Work out the finished part from the listing and answer in its coordinate system (mm). A direction names the side the tool comes from. Coordinates: 2 decimals unless noted, no trailing zeros. Order: outer loops, then holes, each group sorted by start corner. A loop starts at its lowest first (then second) coordinate and runs counter-clockwise, first axis right, second up.
1. Flat-ended cylindrical pins translate along their axes: pin 1 Ø4 at (x, y) = (41.5, -9.5) entering from -Z; pin 2 Ø6 at (y, z) = (-5.5, -31) entering from +X; pin 3 Ø3 at (y, z) = (-10.5, -51.5) entering from -X. Find the tip coordinate at first contact, or state that the pin passes through.
2. Find the intervals of material crossed by probe 1 along X at (y, z) = (2.8, -8); probe 2 along X at (y, z) = (1.4, -62); probe 3 along Z at (x, y) = (7, 2.5), in increasing order.
3. The part is cut by section A-A, the plane z = -62. Give the vertices of the cut face in (x, y).
4. The part is cut by section B-B, the plane z = -41. Give the vertices of the cut face in (x, y).
5. Determine the mould class of faces 4 (the cylindrical face through (25, 2, -37.6)), 5 (the flat face through (35, 4, -32)), 6 (the flat face through (66.05, -6, -11)) for opening direction X: +X half, -X half, draft (parallel to the pull), parting line (faces both ways), or undercut.
6. The part is cut by section C-C, the plane x = 3. Give the vertices of the cut face in (y, z), then the cut area to 3 significant figures.
7. The part is cut by section D-D, the plane y = 2.5. Count the separate pieces of the cut face and the enclosed holes in it, then the cut area to 3 significant figures.
8. A tool of negligible diameter and unlimited length cuts with its end or side. For faces 1 (the flat face through (69, -6, -4)), 2 (the flat face through (36.3, -3, -37)), 3 (the cylindrical face through (9.5, 2, -37.7)), from which of +Z, -Z, +X, -X, +Y, -Y can it reach the whole face along a straight path? Write none if from no direction.
```python
from build123d import *

# Parameters (mm, degrees)
BOSS_EXTRUDE1_DEPTH     = 4
BOSS_EXTRUDE2_DEPTH     = 8.75
SKETCH3_W               = 33.5
SKETCH3_H               = 17.75
BOSS_EXTRUDE3_DEPTH     = 4
SKETCH4_W               = 18.5
SKETCH4_H               = 39.5
CUT_EXTRUDE1_DEPTH      = 4
SKETCH5_W               = 5.5
SKETCH5_H               = 12.75
BOSS_EXTRUDE4_DEPTH     = 4
CUT_EXTRUDE2_DEPTH      = 98.503666598
CUT_EXTRUDE2_DEPTH_BACK = 98.503666598
SKETCH6_R               = 1.25
SKETCH7_R               = 2.5
SKETCH7_R_2             = 1.25
BOSS_EXTRUDE5_DEPTH     = 4
CUT_EXTRUDE3_DEPTH      = 99.106905975
CUT_EXTRUDE3_DEPTH_BACK = 99.106905975
SKETCH8_R               = 1.25
CUT_EXTRUDE4_DEPTH      = 95.88395544
CUT_EXTRUDE4_DEPTH_BACK = 95.88395544
SKETCH9_R               = 1.5
SKETCH11_W              = 32
SKETCH11_H              = 32
SKETCH11_W_2            = 26
SKETCH11_H_2            = 26
BOSS_EXTRUDE6_DEPTH     = 12.75
CUT_EXTRUDE6_DEPTH      = 94.014259659
CUT_EXTRUDE6_DEPTH_BACK = 94.014259659
CUT_EXTRUDE7_DEPTH      = 90.802714324
CUT_EXTRUDE7_DEPTH_BACK = 5


with BuildPart() as part:
    # Sketch1 → Boss-Extrude1 (new body)
    with BuildSketch(Plane(origin=(0, 0, 0), x_dir=(1, 0, 0), z_dir=(0, 1, 0))):
        Polygon((0, 0), (36.55, 0), (36.55, 13.75), (62.05, 13.75), (62.05, 0), (71.55, 0), (71.55, 65), (0, 65), align=None)
    extrude(amount=BOSS_EXTRUDE1_DEPTH)

    # Sketch2 → Boss-Extrude2 (add)
    with BuildSketch(Plane(origin=(0, 0, 0), x_dir=(1, 0, 0), z_dir=(0, 1, 0))):
        Polygon((62.05, 13.75), (62.05, 0), (66.05, 0), (66.05, 17.75), (32.55, 17.75), (32.55, 0), (36.55, 0), (36.55, 13.75), align=None)
    extrude(amount=-BOSS_EXTRUDE2_DEPTH)

    # Sketch3 → Boss-Extrude3 (add)
    with BuildSketch(Plane.XZ.offset(8.75)):
        with Locations((49.3, -8.875)):
            Rectangle(SKETCH3_W, SKETCH3_H)
    extrude(amount=BOSS_EXTRUDE3_DEPTH)

    # Sketch4 → Cut-Extrude1 (cut)
    with BuildSketch(Plane(origin=(0, 4, 0), x_dir=(1, 0, 0), z_dir=(0, 1, 0))):
        with Locations((17.25, 35.25)):
            Rectangle(SKETCH4_W, SKETCH4_H)
    extrude(amount=-CUT_EXTRUDE1_DEPTH, mode=Mode.SUBTRACT)

    # Sketch5 → Boss-Extrude4 (add)
    with BuildSketch(Plane.XY):
        with Locations((29.8, -6.375)):
            Rectangle(SKETCH5_W, SKETCH5_H)
        with Locations((68.8, -6.375)):
            Rectangle(SKETCH5_W, SKETCH5_H)
    extrude(amount=-BOSS_EXTRUDE4_DEPTH)

    # Sketch6 → Cut-Extrude2 (cut, two sides: drawn at the far end of the back side and taken through both)
    with BuildSketch(Plane.XZ.offset(-CUT_EXTRUDE2_DEPTH_BACK)):
        with Locations(Location((7, -13.19, 0), (0, 0, 270))):
            Circle(SKETCH6_R)
        with Locations(Location((27.5, -13.19, 0), (0, 0, 270))):
            Circle(SKETCH6_R)
        with BuildLine():
            ThreePointArc((26.5, -38.44), (27.895284708, -38.875854123), (28.75, -37.69))
            ThreePointArc((28.75, -37.69), (27.895284708, -36.504145877), (26.5, -36.94))
            Line((26.5, -36.94), (26.5, -38.44))
        make_face()
        with BuildLine():
            Line((26.5, -38.44), (26.5, -36.94))
            ThreePointArc((26.5, -36.94), (26.25, -37.69), (26.5, -38.44))
        make_face()
        with BuildLine():
            ThreePointArc((8, -38.44), (8.185854123, -38.085284708), (8.25, -37.69))
            ThreePointArc((8.25, -37.69), (8.185854123, -37.294715292), (8, -36.94))
            Line((8, -36.94), (8, -38.44))
        make_face()
        with BuildLine():
            Line((8, -38.44), (8, -36.94))
            ThreePointArc((8, -36.94), (5.75, -37.69), (8, -38.44))
        make_face()
    extrude(amount=CUT_EXTRUDE2_DEPTH + CUT_EXTRUDE2_DEPTH_BACK, mode=Mode.SUBTRACT)

    # Sketch7 → Boss-Extrude5 (add)
    # profile 1 of 2: a face of its own
    with BuildSketch(Plane.XZ):
        with Locations((7, -37.69)):
            Circle(SKETCH7_R)
        with Locations(Location((7, -37.69, 0), (0, 0, 270))):
            Circle(SKETCH7_R_2, mode=Mode.SUBTRACT)
    # profile 2 of 2: a face of its own
    with BuildSketch(Plane.XZ):
        with Locations((27.5, -37.69)):
            Circle(SKETCH7_R)
        with Locations(Location((27.5, -37.69, 0), (0, 0, 270))):
            Circle(SKETCH7_R_2, mode=Mode.SUBTRACT)
    extrude(amount=-BOSS_EXTRUDE5_DEPTH)

    # Sketch8 → Cut-Extrude3 (cut, two sides: drawn at the far end of the back side and taken through both)
    with BuildSketch(Plane(origin=(0, 4, 0), x_dir=(1, 0, 0), z_dir=(0, 1, 0)).offset(-CUT_EXTRUDE3_DEPTH_BACK)):
        with Locations(Location((3, 62, 0), (0, 0, 90))):
            Circle(SKETCH8_R)
        with Locations(Location((68.55, 62, 0), (0, 0, 90))):
            Circle(SKETCH8_R)
        with Locations(Location((68.55, 8, 0), (0, 0, 90))):
            Circle(SKETCH8_R)
        with Locations(Location((3, 8, 0), (0, 0, 90))):
            Circle(SKETCH8_R)
    extrude(amount=CUT_EXTRUDE3_DEPTH + CUT_EXTRUDE3_DEPTH_BACK, mode=Mode.SUBTRACT)

    # Sketch9 → Cut-Extrude4 (cut, two sides: drawn at the far end of the back side and taken through both)
    with BuildSketch(Plane(origin=(0, 0, -4), x_dir=(-1, 0, 0), z_dir=(0, 0, -1)).offset(-CUT_EXTRUDE4_DEPTH_BACK)):
        with Locations((-68.8, -9.75)):
            Circle(SKETCH9_R)
        with Locations((-29.8, -9.75)):
            Circle(SKETCH9_R)
    extrude(amount=CUT_EXTRUDE4_DEPTH + CUT_EXTRUDE4_DEPTH_BACK, mode=Mode.SUBTRACT)

    # Sketch11 → Boss-Extrude6 (add)
    with BuildSketch(Plane.XZ):
        with Locations((49.3, -36.75)):
            Rectangle(SKETCH11_W, SKETCH11_H)
        with Locations((49.3, -36.75)):
            Rectangle(SKETCH11_W_2, SKETCH11_H_2, mode=Mode.SUBTRACT)
    extrude(amount=BOSS_EXTRUDE6_DEPTH)

    # Sketch12 → Cut-Extrude6 (cut, two sides: drawn at the far end of the back side and taken through both)
    with BuildSketch(Plane(origin=(65.3, 0, 0), x_dir=(0, 0, -1), z_dir=(1, 0, 0)).offset(-CUT_EXTRUDE6_DEPTH_BACK)):
        with BuildLine():
            ThreePointArc((39.25, -7), (38.517766953, -5.232233047), (36.75, -4.5))
            Line((36.75, -4.5), (36.75, -9.5))
            ThreePointArc((36.75, -9.5), (38.517766953, -8.767766953), (39.25, -7))
        make_face()
        with BuildLine():
            Line((36.75, -9.5), (36.75, -4.5))
            ThreePointArc((36.75, -4.5), (34.25, -7), (36.75, -9.5))
        make_face()
    extrude(amount=CUT_EXTRUDE6_DEPTH + CUT_EXTRUDE6_DEPTH_BACK, mode=Mode.SUBTRACT)

    # Sketch13 → Cut-Extrude7 (cut, two sides: drawn at the far end of the back side and taken through both)
    with BuildSketch(Plane(origin=(0, 0, -52.75), x_dir=(-1, 0, 0), z_dir=(0, 0, -1)).offset(-CUT_EXTRUDE7_DEPTH_BACK)):
        with BuildLine():
            ThreePointArc((-46.8, -7), (-47.532233047, -5.232233047), (-49.3, -4.5))
            Line((-49.3, -4.5), (-49.3, -9.5))
            ThreePointArc((-49.3, -9.5), (-47.532233047, -8.767766953), (-46.8, -7))
        make_face()
        with BuildLine():
            Line((-49.3, -9.5), (-49.3, -4.5))
            ThreePointArc((-49.3, -4.5), (-51.8, -7), (-49.3, -9.5))
        make_face()
    extrude(amount=CUT_EXTRUDE7_DEPTH + CUT_EXTRUDE7_DEPTH_BACK, mode=Mode.SUBTRACT)


solid = part.part
```
Geometry says:
1. pin 1: stops at z = -52.75
1. pin 2: stops at x = 65.3
1. pin 3: stops at x = 33.3
2. probe 1: x = 0 to 1.75, 4.25 to 36.55, 62.05 to 67.3, 69.8 to 71.55
2. probe 2: x = 0 to 1.75, 4.25 to 67.3, 69.8 to 71.55
2. probe 3: z = -65 to -38.94, -36.44 to -14.44, -11.94 to 0
3. outline: (0, 0) - (1.75, 0) - (1.75, 4) - (0, 4) - close; (4.25, 0) - (67.3, 0) - (67.3, 4) - (4.25, 4) - close; (69.8, 0) - (71.55, 0) - (71.55, 4) - (69.8, 4) - close
4. outline: (0, 0) - (8, 0) - (8, 4) - (0, 4) - close; (26.5, 0) - (33.3, 0) - (33.3, -12.75) - (36.3, -12.75) - (36.3, 0) - (62.3, 0) - (62.3, -12.75) - (65.3, -12.75) - (65.3, 0) - (71.55, 0) - (71.55, 4) - (26.5, 4) - close
5. face 4: undercut
5. face 5: draft
5. face 6: +X half
6. outline: (0, -65) - (4, -65) - (4, -63.25) - (0, -63.25) - close; (0, -60.75) - (4, -60.75) - (4, -9.25) - (0, -9.25) - close; (0, -6.75) - (4, -6.75) - (4, 0) - (0, 0) - close
6. area: 240 mm2
7. separate pieces: 1
7. enclosed holes: 9
7. area: 3,540 mm2
8. face 1: -Z, +X, -Y
8. face 2: -Y
8. face 3: +Y, -Y
